Verification items for the finished model (mm, model axes). Face numbers are marked on the shaded views. A direction names the side the tool comes from. Give positions to 0.01 mm unless a question says otherwise; leave off trailing zeros. Order: outer loops, then holes, each group sorted by start corner. A loop starts at its lowest first (then second) coordinate and runs counter-clockwise, first axis right, second up.
from build123d import *

# Parameters (mm, degrees)
F1_DEPTH  = 38.1
F2_W      = 25.4
F2_H      = 38.1
F3_DEPTH  = 25.4
F4_R      = 6.35
F5_DEPTH  = 12.7
F7_DEPTH  = 12.7
F8_W      = 12.7
F8_H      = 12.7
F9_DEPTH  = 12.7
F11_DEPTH = 12.7
F12_R     = 1.5875
F13_DEPTH = 6.35


with BuildPart() as f1:
    # F0 (on Front) → F1 (new body)
    with BuildSketch(Plane.XZ):
        Polygon((-17.457331, 44.45), (-42.857331, 44.45), (-42.857331, 0), (26.992669, 0), (26.992669, 6.35), (-17.457331, 6.35), align=None)
    extrude(amount=F1_DEPTH)

    # F2 (on face) → F3 (cut)
    with BuildSketch(Plane.XZ.offset(38.1)):
        with Locations((-30.157331, 25.4)):
            Rectangle(F2_W, F2_H)
    extrude(amount=-F3_DEPTH, mode=Mode.SUBTRACT)

    # F4 (on face) → F5 (cut)
    with BuildSketch(Plane.XZ.offset(12.7)):
        with Locations((-30.157331, 31.75)):
            Circle(F4_R)
    extrude(amount=-F5_DEPTH, mode=Mode.SUBTRACT)

    # F6 (on face) → F7 (cut)
    with BuildSketch(Plane.XZ.offset(12.7)):
        with BuildLine():
            ThreePointArc((-42.857331, 31.75), (-39.137587, 40.730256), (-30.157331, 44.45))
            Line((-30.157331, 44.45), (-42.857331, 44.45))
            Line((-42.857331, 44.45), (-42.857331, 31.75))
        make_face()
        with BuildLine():
            Line((-17.457331, 44.45), (-30.157331, 44.45))
            ThreePointArc((-30.157331, 44.45), (-21.177075, 40.730256), (-17.457331, 31.75))
            Line((-17.457331, 31.75), (-17.457331, 44.45))
        make_face()
    extrude(amount=-F7_DEPTH, mode=Mode.SUBTRACT)

    # F8 (on face) → F9 (join)
    with BuildSketch(Plane.XZ.offset(12.7)):
        with Locations((-11.107331, 12.7)):
            Rectangle(F8_W, F8_H)
    extrude(amount=-F9_DEPTH)

    # F10 (on face) → F11 (cut)
    with BuildSketch(Plane.XZ.offset(12.7)):
        with BuildLine():
            Line((-4.757331, 19.05), (-17.457331, 19.05))
            ThreePointArc((-17.457331, 19.05), (-13.737587, 10.069744), (-4.757331, 6.35))
            Line((-4.757331, 6.35), (-4.757331, 19.05))
        make_face()
    extrude(amount=-F11_DEPTH, mode=Mode.SUBTRACT)

    # F12 (on face) → F13 (cut)
    with BuildSketch(Plane.XY.offset(6.35)):
        with Locations((-33.332331, -28.575)):
            Circle(F12_R)
        with Locations((17.467669, -28.575)):
            Circle(F12_R)
        with Locations((17.467669, -9.525)):
            Circle(F12_R)
    extrude(amount=-F13_DEPTH, mode=Mode.SUBTRACT)


solid = f1.part
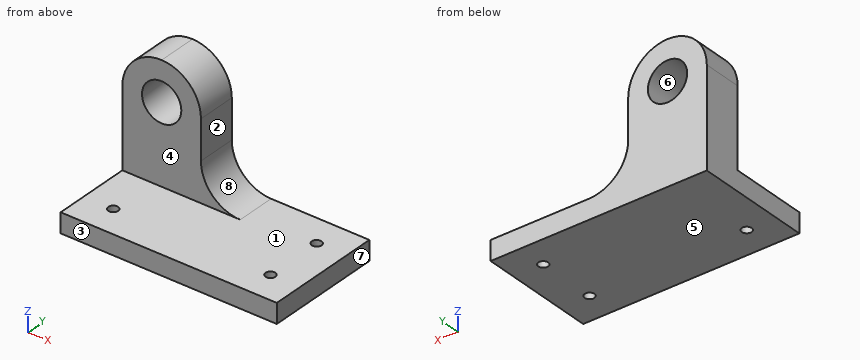
(1) Section check C-C, the plane y = -22. Enter the section's corners in (x, z), then the cut area to 3 significant figures.
Solved:
outline: (-42.86, 0) - (26.99, 0) - (26.99, 6.35) - (-42.86, 6.35) - close
area: 444 mm2
(2) Go/stop test with flat-tipped pins: pin 1 (3 mm diameter, centred on x = 8, y = -19, fed in from +Z); pin 2 (6.5 mm diameter, centred on y = -5, z = 28.5, fed in from +X); pin 3 (19 mm diameter, centred on x = -17.5, z = 24.5, fed in from -Y). Record where each tip stops, or that it passes through.
Solved:
pin 1: stops at z = 6.35
pin 2: stops at x = -17.46
pin 3: stops at y = -12.7
(3) Scan lines: line 1 (Z direction, x = -38, y = -23.5); line 2 (Y direction, x = -26, z = 22.5). Record each from-to range of solid material in increasing order.
Solved:
line 1: z = 0 to 6.35
line 2: y = -12.7 to 0
(4) Set-up check for the marked faces 1, 2, 3 and 4: record each of +Z, -Z, +X, -X, +Y, -Y from which the full face is reachable in a straight line by a thin tool's end or side.
Solved:
face 1: +Z, +X, -Y
face 2: +Z, +X, +Y, -Y
face 3: +Z, -Z, +X, -X, -Y
face 4: +Z, +X, -X, -Y
(5) Section check B-B, the plane z = 35. Enter the section's corners in (x, y), then the cut area to 3 significant figures.
Solved:
outline: (-42.43, -12.7) - (-35.61, -12.7) - (-35.61, 0) - (-42.43, 0) - close; (-24.7, -12.7) - (-17.88, -12.7) - (-17.88, 0) - (-24.7, 0) - close
area: 173 mm2
(6) Section check A-A, the plane x = -25.5. Enter the section's corners in (y, z).
Solved:
outline: (-38.1, 0) - (0, 0) - (0, 27.43) - (-12.7, 27.43) - (-12.7, 6.35) - (-38.1, 6.35) - close; (-12.7, 36.07) - (0, 36.07) - (0, 43.57) - (-12.7, 43.57) - close
(7) Section check D-D, the plane x = 7.5. Enter the section's corners in (y, z), then the cut area to 3 significant figures.
Solved:
outline: (-38.1, 0) - (0, 0) - (0, 6.35) - (-38.1, 6.35) - close
area: 242 mm2
(8) Release check for a two-part mould opening along Z. For the marked faces 5, 6, 7 and 8 record: pulls with the +Z half, pulls with the -Z half, needs draft (parallel to the pull), parting line crosses it, or undercut.
Solved:
face 5: pulls with the -Z half
face 6: undercut
face 7: needs draft
face 8: pulls with the +Z half
